```python
from build123d import *

# Parameters (mm, degrees)
F0_W     = 50.8
F0_H     = 50.8
F1_DEPTH = 25.4
F2_DEPTH = 25.4


# Not quite as in the source:
# - a feature names something its author has since deleted; it is built from what else it names


with BuildPart() as f1:
    # F0 (on Top) → F1 (new body)
    with BuildSketch(Plane.XY):
        with Locations((25.4, -16.6914236449)):
            Rectangle(F0_W, F0_H)
        Polygon((28.5474364771, -8.2873642427), (34.2667401254, -18.5540249534), (26.2699275792, -27.1659785919), (15.6083219757, -22.2217979392), (17.0158998843, -10.5541726109), align=None, mode=Mode.SUBTRACT)
        Polygon((35.5715639889, 7.9258885235), (48.6309623563, -0.3860413606), (34.9029207385, -7.5398471628), align=None, mode=Mode.SUBTRACT)
    extrude(amount=F1_DEPTH)

    # F0 (on Top) → F2 (join)
    with BuildSketch(Plane.XY):
        with Locations((25.4, -16.6914236449)):
            Rectangle(F0_W, F0_H)
        Polygon((28.5474364771, -8.2873642427), (34.2667401254, -18.5540249534), (26.2699275792, -27.1659785919), (15.6083219757, -22.2217979392), (17.0158998843, -10.5541726109), align=None, mode=Mode.SUBTRACT)
        Polygon((35.5715639889, 7.9258885235), (48.6309623563, -0.3860413606), (34.9029207385, -7.5398471628), align=None, mode=Mode.SUBTRACT)
    extrude(amount=F2_DEPTH)


solid = f1.part
```
Check sheet for the modelled part. Datum: model origin and axes. Units: mm. A direction names the side the tool comes from. Round coordinates to 2 decimals unless told otherwise and drop trailing zeros. Order: outer loops, then holes, each group sorted by start corner. A loop starts at its lowest first (then second) coordinate and runs counter-clockwise, first axis right, second up. Notation, with made-up numbers: (-25.75, 74) -> (-6.75, 74) arc R21 cw to (-6.75, 110) -> close; hole circle Ø9 at (9.25, -3.5). An arc over 180 degrees is marked (long way). One line per item, written item: value. Start each with the question number.
Q1. Cross-section at B-B (x = 44.5). Record the boundary of the cut face in (y, z).
Q2. Cross-section at A-A (z = 23.75). Record the boundary of the cut face in (x, y), and give its area (3 significant figures).
Q3. Thickness scan on line 1 (Y direction, x = 48.5, z = 22.25); line 2 (Y direction, x = 30, z = 17.5); line 3 (X direction, y = -23.5, z = 20.25). Record the ranges inside material, lowest first.
Q4. Cross-section at C-C (y = -17). Record the boundary of the cut face in (x, z), and give its area (3 significant figures).
Q5. Mould release check, pull along X, two halves, no side actions. Record for faces 1 (the face through (21.014, -24.728, 12.522)), 2 (the face through (50.8, -17, 13)), 3 (the face through (0, -17, 13)), 4 (the face through (25, -42.091, 13)): pulls with the +X half, pulls with the -X half, needs draft (parallel to the pull), parting line crosses it, or undercut.
Q6. Gauge pin test, flat end, axial feed: pin 1 Ø6 at (y, z) = (-16.5, 10.5) entering from -X. Record the tip position at first contact, or that the pin passes through.
Q7. Set-up check for faces 5 (the face through (42.01, 3.83, 12.52)), 6 (the face through (31, -11, 0)): record each of +Z, -Z, +X, -X, +Y, -Y from which the full face is reachable in a straight line by a thin tool's end or side.
Completed:
1. outline: (-42.09, 0) -> (-2.54, 0) -> (-2.54, 25.4) -> (-42.09, 25.4) -> close; (2.24, 0) -> (8.71, 0) -> (8.71, 25.4) -> (2.24, 25.4) -> close
2. outline: (0, -42.09) -> (50.8, -42.09) -> (50.8, 8.71) -> (0, 8.71) -> close; hole (15.61, -22.22) -> (26.27, -27.17) -> (34.27, -18.55) -> (28.55, -8.29) -> (17.02, -10.55) -> close; hole (34.9, -7.54) -> (48.63, -0.39) -> (35.57, 7.93) -> close
2. area: 2,240 mm²
3. line 1: y = -42.09 to -0.45, -0.3 to 8.71
3. line 2: y = -42.09 to -23.15, -10.89 to 8.71
3. line 3: x = 0 to 18.36, 29.67 to 50.8
4. outline: (0, 0) -> (16.24, 0) -> (16.24, 25.4) -> (0, 25.4) -> close; (33.4, 0) -> (50.8, 0) -> (50.8, 25.4) -> (33.4, 25.4) -> close
4. area: 854 mm²
5. face 1: undercut
5. face 2: pulls with the +X half
5. face 3: pulls with the -X half
5. face 4: needs draft
6. pin 1: stops at x = 0
7. face 5: +Z, -Z
7. face 6: -Z, +X, -X, +Y, -Y
